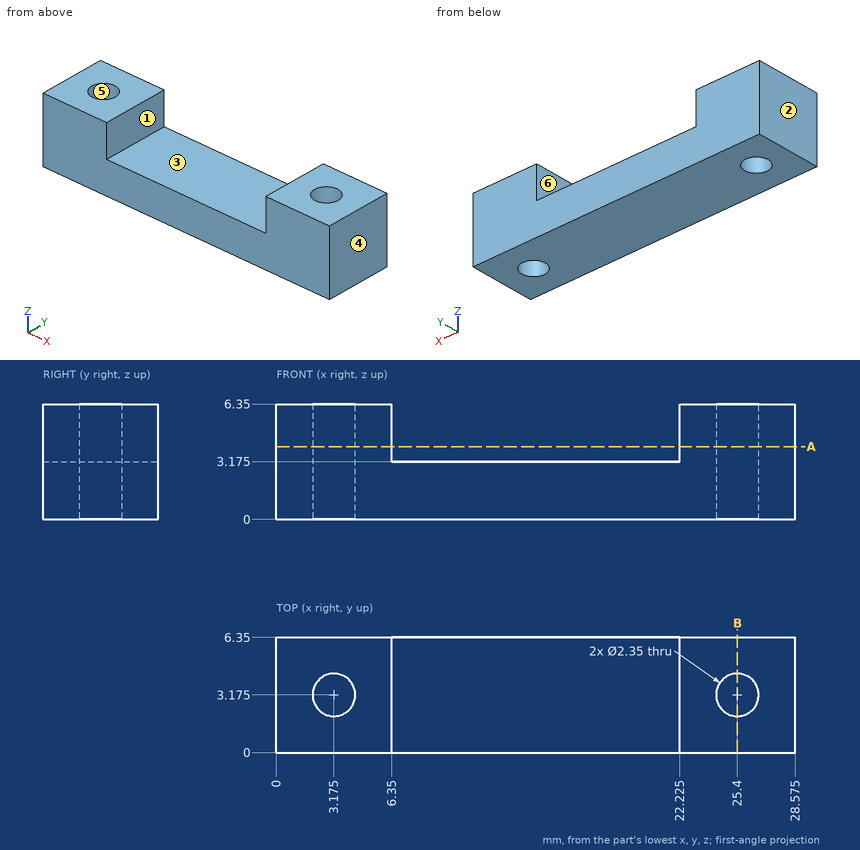
Geometry check sheet. Reference: drawing and pictorial views, mm from the part's lowest x, y, z. A direction names the side the tool comes from. Coordinates: 2 decimals unless noted, no trailing zeros. Write each loop counter-clockwise with the first axis right and the second up, starting at its lowest first coordinate (ties: lowest second). Pieces come first, ordered by that corner, then holes. Notation, with made-up numbers: M -9.5,38 L 6.5,38 A9 ccw 6.5,50 Z; hole C 72.25,52.25 d8. An arc over 180 degrees is marked long. Use one line per item in the form item = value.
Item 1: Material ranges on L1, parallel to Y at x = 25.4, z = 5; L2, parallel to X at y = 2.5, z = 2.25 (1 decimal); L3, parallel to Z at x = 19, y = 1.5 (1 decimal), recorded low to high. Write a range as from..to.
Answer below:
L1 = 0..2, 4.35..6.35
L2 = 0..2.2, 4.1..24.4, 26.4..28.6
L3 = 0..3.2
Item 2: Sectioned sample at B-B, the plane x = 25.4. Record the cut outline in (y, z), and give its area (3 significant figures).
Answer below:
outline = M 0,0 L 2,0 L 2,6.35 L 0,6.35 Z; M 4.35,0 L 6.35,0 L 6.35,6.35 L 4.35,6.35 Z
area = 25.4 mm^2
Item 3: Sectioned sample at A-A, the plane z = 4. State how many separate pieces and enclosed holes the cut face has.
Answer below:
separate_pieces = 2
enclosed_holes = 2
Item 4: Release check for a two-part mould opening along X. For the marked faces 1, 2, 3 and 4 record: pulls with the +X half, pulls with the -X half, needs draft (parallel to the pull), parting line crosses it, or undercut.
Answer below:
face_1 = undercut
face_2 = pulls with the -X half
face_3 = undercut
face_4 = pulls with the +X half
Item 5: Set-up check for the marked faces 5 and 6: record each of +Z, -Z, +X, -X, +Y, -Y from which the full face is reachable in a straight line by a thin tool's end or side.
Answer below:
face_5 = +Z, -Z
face_6 = +Z, +Y, -Y
